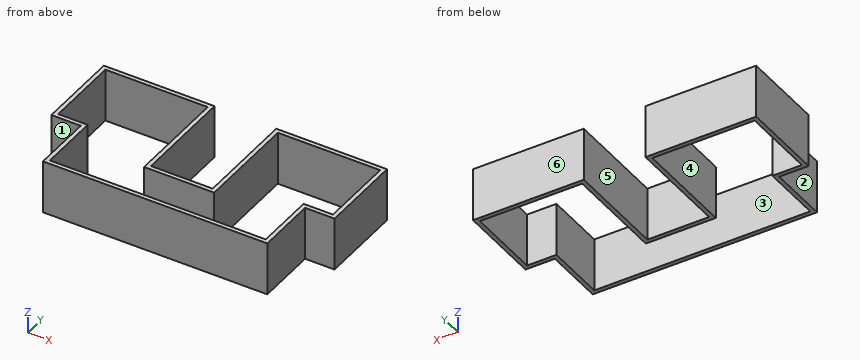
from build123d import *

# Parameters (mm, degrees)
BOSS_EXTRUDE1_DEPTH = 38.1
SHELL2_T            = -3


with BuildPart() as part:
    # Sketch1 → Boss-Extrude1 (new body)
    with BuildSketch(Plane.XY):
        Polygon((80, 0), (-80, 0), (-80, 43.25), (-101, 43.25), (-101, 103.25), (-22.006, 103.25), (-22.006, 30.441483681), (22.006, 30.441483681), (22.006, 103.25), (101, 103.25), (101, 43.25), (80, 43.25), align=None)
    extrude(amount=BOSS_EXTRUDE1_DEPTH)

    # Shell2
    shell2_openings = [part.faces().sort_by_distance(p)[0] for p in [
        (0, 2.268580228, 38.1),
        (0, 2.268580228, 0),
    ]]
    offset(amount=SHELL2_T, openings=shell2_openings, kind=Kind.INTERSECTION)


solid = part.part
Model file for the job. Use its own axes, mm. Face numbers are marked on the shaded views. A direction names the side the tool comes from. Round coordinates to 2 decimals unless told otherwise and drop trailing zeros. Order: outer loops, then holes, each group sorted by start corner. A loop starts at its lowest first (then second) coordinate and runs counter-clockwise, first axis right, second up. Notation, with made-up numbers: M -39,-25.5 L -18,-25.5 A14 cw -18,-14.5 Z; hole C 64.25,87 d4. An arc over 180 degrees is marked long. Write each question's results on one line, items separated by ' | '. Start each with the question number.
(1) Drop flat-ended pins along their axis: pin 1 (19 mm diameter, centred on y = 27, z = 22.5, fed in from -X); pin 2 (4 mm diameter, centred on y = 25.5, z = 19.5, fed in from +X); pin 3 (11.5 mm diameter, centred on x = 3.5, z = 19, fed in from +Y). Give the stop position or say it passes through.
(2) Probe probe 1 along X at (y, z) = (72, 8.5); probe 2 along X at (y, z) = (39.5, 32); probe 3 along Y at (x, z) = (51, 10). List the from-to ranges inside material, lowest first. Write a range as from..to.
(3) Which spindle directions (+Z, -Z, +X, -X, +Y, -Y) get a long thin tool onto all of the face, cutting with end or side? Do the marked faces 4, 5 and 6. Say none if no direction does.
(4) Saw through at B-B, the plane x = -56.5. Give the cut face in (y, z), then the cut area to 3 significant figures.
(5) Saw through at A-A, the plane y = 41. Give the cut face in (x, z), then the cut area to 3 significant figures.
(6) Saw through at D-D, the plane z = 5.5. Give the cut face in (x, y).
(7) Two-plate mould, pull along Y, no slides. Class the marked faces 1, 2 and 3: pulls with the +Y half, pulls with the -Y half, needs draft (parallel to the pull), parting line crosses it, or undercut.
(8) Saw through at C-C, the plane y = 19.5. Give the cut face in (x, z), then the cut area to 3 significant figures.
Established:
1) pin 1: stops at x = -80 | pin 2: stops at x = 80 | pin 3: stops at y = 30.44
2) probe 1: x = -101..-98, -25.01..-22.01, 22.01..25.01, 98..101 | probe 2: x = -80..-77, -25.01..-22.01, 22.01..25.01, 77..80 | probe 3: y = 0..3, 100.25..103.25
3) face 4: +Z, -Z | face 5: +Z, -Z, +Y | face 6: +Z, -Z, +X, -X, +Y
4) outline: M 0,0 L 3,0 L 3,38.1 L 0,38.1 Z; M 100.25,0 L 103.25,0 L 103.25,38.1 L 100.25,38.1 Z | area: 229 mm^2
5) outline: M -80,0 L -77,0 L -77,38.1 L -80,38.1 Z; M -25.01,0 L -22.01,0 L -22.01,38.1 L -25.01,38.1 Z; M 22.01,0 L 25.01,0 L 25.01,38.1 L 22.01,38.1 Z; M 77,0 L 80,0 L 80,38.1 L 77,38.1 Z | area: 457 mm^2
6) outline: M -101,43.25 L -80,43.25 L -80,0 L 80,0 L 80,43.25 L 101,43.25 L 101,103.25 L 22.01,103.25 L 22.01,30.44 L -22.01,30.44 L -22.01,103.25 L -101,103.25 Z; hole M -98,46.25 L -77,46.25 L -77,3 L 77,3 L 77,46.25 L 98,46.25 L 98,100.25 L 25.01,100.25 L 25.01,27.44 L -25.01,27.44 L -25.01,100.25 L -98,100.25 Z
7) face 1: pulls with the -Y half | face 2: needs draft | face 3: undercut
8) outline: M -80,0 L -77,0 L -77,38.1 L -80,38.1 Z; M 77,0 L 80,0 L 80,38.1 L 77,38.1 Z | area: 229 mm^2
